Verification items for the finished model (mm, model axes). A direction names the side the tool comes from. Give positions to 0.01 mm unless a question says otherwise; leave off trailing zeros. Order: outer loops, then holes, each group sorted by start corner. A loop starts at its lowest first (then second) coordinate and runs counter-clockwise, first axis right, second up. Notation, with made-up numbers: (62.25, 79.25) -> (89.25, 79.25) arc R33 ccw to (89.25, 110.25) -> close; hole circle Ø3 at (77, -38.75). An arc over 180 degrees is marked (long way). Return JSON: item names as keys, results as strings. Group by question number.
(1) Cross-section at C-C on y = -56. Enter the section's corners in (x, z), then the cut area to 3 significant figures.
(2) Cross-section at B-B on x = 61. Enter the section's corners in (y, z).
(3) Thickness scan on line 1 along X through (y, z) = (-81, -66.5); line 2 along Y through (x, z) = (95, 34); line 3 along Z through (x, y) = (214, -88). Record the ranges inside material, lowest first.
(4) Cross-section at A-A on z = 114. Enter the section's corners in (x, y), then the cut area to 3 significant figures.
(5) Tool access check on faces 1 (the face through (215.9, -83, -2)), 2 (the face through (209.55, -83, -2)). Record the directions out of +Z, -Z, +X, -X, +Y, -Y that give a thin tool (end or side, any length) a straight path to the whole face; none if there is none.
(6) Release check for a two-part mould opening along Y. For faces 3 (the face through (2, -12.7, -2)), 4 (the face through (212.769, -92.774, 0.86)), 5 (the face through (50, -9, -177.8)), 6 (the face through (212.769, -91.315, 142.849)) record: pulls with the +Y half, pulls with the -Y half, needs draft (parallel to the pull), parting line crosses it, or undercut.
(7) Depth check by flat-ended pin: pin 1 Ø5 at (y, z) = (-69.5, -118) entering from +X; pin 2 Ø7.5 at (y, z) = (-94.5, 15) entering from -X; pin 3 Ø5 at (x, z) = (206.5, 61) entering from -Y. Enter the tip coordinate at first touch or a pass-through.
from build123d import *

# Parameters (mm, degrees)
BOSS_EXTRUDE1_DEPTH      = 177.8
BOSS_EXTRUDE1_DEPTH_BACK = 177.8
SKETCH2_W                = 6.35
SKETCH2_H                = 355.6
BOSS_EXTRUDE2_DEPTH      = 25.4
SKETCH3_R                = 3.96875
CUT_EXTRUDE1_DEPTH       = 25.4


with BuildPart() as part:
    # Sketch1 → Boss-Extrude1 (new, two sides: drawn at the far end of the back side and taken through both)
    with BuildSketch(Plane.XY.offset(-BOSS_EXTRUDE1_DEPTH_BACK)):
        with BuildLine():
            Line((-139.7, 0), (139.7, 0))
            ThreePointArc((139.7, 0), (193.581536726, -22.318463274), (215.9, -76.2))
            Line((215.9, -76.2), (203.2, -76.2))
            ThreePointArc((203.2, -76.2), (184.601280605, -31.298719395), (139.7, -12.7))
            Line((139.7, -12.7), (-139.7, -12.7))
            Line((-139.7, -12.7), (-139.7, 0))
        make_face()
    extrude(amount=BOSS_EXTRUDE1_DEPTH + BOSS_EXTRUDE1_DEPTH_BACK)

    # Sketch2 → Boss-Extrude2 (add)
    with BuildSketch(Plane.XZ.offset(76.2)):
        with Locations((212.725, 0)):
            Rectangle(SKETCH2_W, SKETCH2_H)
    extrude(amount=BOSS_EXTRUDE2_DEPTH)

    # Sketch3 → Cut-Extrude1 (cut)
    with BuildSketch(Plane(origin=(215.9, 0, 0), x_dir=(0, 0, -1), z_dir=(1, 0, 0))):
        with Locations((-139.7, -88.9)):
            Circle(SKETCH3_R)
        with Locations((0, -88.9)):
            Circle(SKETCH3_R)
        with Locations((139.7, -88.9)):
            Circle(SKETCH3_R)
    extrude(amount=-CUT_EXTRUDE1_DEPTH, mode=Mode.SUBTRACT)


solid = part.part
Verdict:
{
 "1": {"outline": "(199.9, -177.8) -> (213.17, -177.8) -> (213.17, 177.8) -> (199.9, 177.8) -> close", "area": "4,720 mm²"},
 "2": {"outline": "(-12.7, -177.8) -> (0, -177.8) -> (0, 177.8) -> (-12.7, 177.8) -> close"},
 "3": {"line 1": "209.55 to 215.9", "line 2": "-12.7 to 0", "line 3": "-177.8 to -143.57, -135.83 to -3.87, 3.87 to 135.83, 143.57 to 177.8"},
 "4": {"outline": "(-139.7, -12.7) -> (139.7, -12.7) arc R63.5 cw to (203.2, -76.2) -> (209.55, -76.2) -> (209.55, -101.6) -> (215.9, -101.6) -> (215.9, -76.2) arc R76.2 ccw to (139.7, 0) -> (-139.7, 0) -> close", "area": "5,100 mm²"},
 "5": {"face 1": "+Z, -Z, +X, +Y, -Y", "face 2": "+Z, -Z, -X, -Y"},
 "6": {"face 3": "pulls with the -Y half", "face 4": "undercut", "face 5": "needs draft", "face 6": "undercut"},
 "7": {"pin 1": "x = 215.78", "pin 2": "x = 209.55", "pin 3": "y = -76.2"}
}
